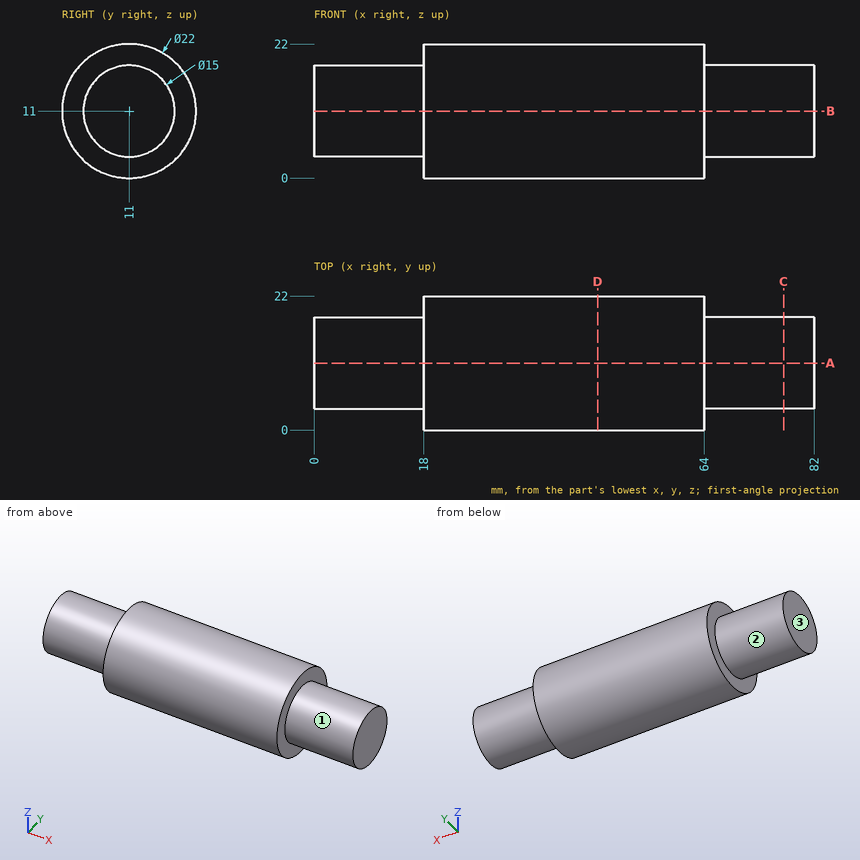
Here's the drawing with two shaded views (mm, measured from the low corner). I have some questions. A direction names the side the tool comes from. Round coordinates to 2 decimals unless told otherwise and drop trailing zeros. Order: outer loops, then holes, each group sorted by start corner. A loop starts at its lowest first (then second) coordinate and runs counter-clockwise, first axis right, second up. Notation, with made-up numbers: (-9.5, -22) -> (25.5, -22) arc R22 cw to (25.5, -9) -> close; hole circle Ø3 at (56.25, 51). An arc over 180 degrees is marked (long way). Write each question's results on one line, items separated by ' | '. Start each with the question number.
Item 1: If we section it at A-A, the plane y = 11: Write out the boundary of the cut face in (x, z).
Item 2: Please list where these lines run through material, in increasing order: L1, parallel to Z at x = 49, y = 11.5; L2, parallel to X at y = 5.75, z = 20.25; L3, parallel to Y at x = 47.5, z = 5.75.
Item 3: If we section it at D-D, the plane x = 46.5: Write out the boundary of the cut face in (y, z).
Item 4: Will these pins go through, and if not, where does the flat tip stop? pin 1 (1 mm diameter, centred on y = 17, z = 19, fed in from +X); pin 2 (12 mm diameter, centred on y = 15, z = 18.5, fed in from -X); pin 3 (4 mm diameter, centred on x = 64.5, y = 14, fed in from +Z); pin 4 (1 mm diameter, centred on x = 47, z = 17.5, fed in from -Y).
Item 5: Which directions (+Z, -Z, +X, -X, +Y, -Y) give clear straight access to the entire face, cutting with the end or side of a thin tool? Please do the marked faces 1, 2 and 3.
Item 6: If we section it at C-C, the plane x = 77: Write out the boundary of the cut face in (y, z), then the cut area to 3 significant figures.
Results:
1) outline: (0, 3.5) -> (18, 3.5) -> (18, 0) -> (64, 0) -> (64, 3.5) -> (82, 3.5) -> (82, 18.5) -> (64, 18.5) -> (64, 22) -> (18, 22) -> (18, 18.5) -> (0, 18.5) -> close
2) L1: z = 0.01 to 21.99 | L2: x = 18 to 64 | L3: y = 1.33 to 20.67
3) outline: circle Ø22 at (11, 11)
4) pin 1: stops at x = 64 | pin 2: stops at x = 0 | pin 3: stops at z = 21.95 | pin 4: stops at y = 1.78
5) face 1: +X | face 2: -X | face 3: +Z, -Z, -X, +Y, -Y
6) outline: circle Ø15 at (11, 11) | area: 177 mm2
